Here's how the part is built. I have some questions about the finished solid (model axes, mm). A direction names the side the tool comes from. Round coordinates to 2 decimals unless told otherwise and drop trailing zeros. Write each loop counter-clockwise with the first axis right and the second up, starting at its lowest first coordinate (ties: lowest second). Pieces come first, ordered by that corner, then holes. Notation, with made-up numbers: (6.25, 51.25) -> (27.25, 51.25) arc R20 cw to (27.25, 76.25) -> close; hole circle Ø4 at (82, 75.25). An arc over 180 degrees is marked (long way). Put each result on its own line as item: value. Start each with the question number.
1. Suppose I cut it at B-B (z = 58). Please give me the cut outline in (x, y).
2. For pin 1 (0.5 mm diameter, centred on x = 0.5, z = -26, fed in from -Y), with a flat end and sliding along its axis, tell me the tip position at first contact or that it passes through.
3. Which directions (+Z, -Z, +X, -X, +Y, -Y) give clear straight access to the entire face, cutting with the end or side of a thin tool? Please do faces 1 (the face through (0.8, 126.57, 160.9)), 2 (the face through (0.78, -10.79, 128.81)).
4. I need wall thicknesses on probe 1 along Z at (x, y) = (1.25, 8.5); probe 2 along Y at (x, z) = (0.25, -10.5); probe 3 along Y at (x, z) = (0.35, -2). Which ranges of each line are inside material? Lowest first, please. Write a range as from..to.
5. We'd pull the mould along Z, two halves only. Please class faces 3 (the face through (0.8, 200.01, 137.73)), 4 (the face through (1.588, 94, 2)), 5 (the face through (0.805, 183.13, 118.068)): +Z half, -Z half, draft (parallel to the pull), parting line (faces both ways), or undercut.
6. Suppose I cut it at C-C (y = 155). Please give me the cut outline in (x, z).
7. Suppose I cut it at A-A (x = 0.7). Count the separate pieces of the cut face and the enclosed holes in it, then the cut area to 3 significant figures.
Autodesk Inventor part; units mm, degrees
ref_plane "YZ Plane" through (0, 0, 0) normal (1, 0, 0) x (0, 1, 0)
ref_plane "XZ Plane" through (0, 0, 0) normal (0, 1, 0) x (-1, 0, 0)
ref_plane "XY Plane" through (0, 0, 0) normal (0, 0, 1) x (1, 0, 0)
sketch "Sketch1" plane through (0, 0, 0) normal (1, 0, 0) x (0, 1, 0)
  line L0 (-12.7, -177.8) -> (12.7, -177.8)
  line L1 (12.7, -177.8) -> (12.7, 177.8)
  line L2 (12.7, 177.8) -> (-12.7, 177.8)
  line L3 (-12.7, 177.8) -> (-12.7, -177.8)
  line L4 (-12.7, -177.8) -> (12.7, 177.8) construction
  line L5 (12.7, -177.8) -> (-12.7, 177.8) construction
  line L6 (12.7, -101.6) -> (12.7, 177.8)
  line L7 (12.7, 177.8) -> (25.4, 177.8)
  line L8 (25.4, 177.8) -> (25.4, -177.8)
  line L9 (25.4, -177.8) -> (12.7, -177.8)
  line L10 (12.7, -177.8) -> (12.7, 177.8)
  line L11 (25.4, 177.8) -> (203.2, 177.8)
  line L12 (203.2, 177.8) -> (203.2, -177.8)
  line L13 (203.2, -177.8) -> (25.4, -177.8)
  line L14 (25.4, -177.8) -> (25.4, 177.8)
  circle A0 centre (41.275, -161.925) radius 15.875
  circle A1 centre (187.325, -59.6597) radius 15.875
  line L15 (41.275, -161.925) -> (203.2, -48.5439)
  line L16 (41.275, -161.925) -> (238.9489, -161.925) construction
  line L17 (196.4305, -72.6637) -> (50.3805, -174.929)
  circle A2 centre (187.325, -59.6597) radius 10.9537
  circle A3 centre (41.275, -161.925) radius 10.9538
  point P0 (0, 0)
  point P1 (203.2, -59.6597)
  point P2 (41.275, -177.8)
  dimension "d7" = 31.75
  dimension "d8" = 31.75
  dimension "d0" = 25.4
  dimension "d1" = 355.6
  dimension "d4" = 12.7
  dimension "d5" = 177.8
  dimension "d6" = 355.6
  dimension "d9" = 35
  dimension "d10" = 21.9075
  dimension "d11" = 21.9075
extrude "Extrusion1" add sketch "Sketch1" along normal blind 1.5875 contours L3 L2 L1 L0 | L1 L7 L8 L9 | L8 A0 L13 | L8 L11 L12 L15 A1 A0 | A0 | L15 A1 L17 A0 | L15 A2 A1 | A1 L15 A2 | A1 L15 L12
sketch "Sketch2" plane through (1.5875, 0, 0) normal (1, 0, 0) x (0, 0, -1)
  line L0 (-177.8, -12.7) -> (177.8, -12.7)
  line L1 (-127, -12.7) -> (127, -12.7)
  line L2 (127, -12.7) -> (127, 25.4)
  line L3 (127, 25.4) -> (-127, 25.4)
  line L4 (-127, 25.4) -> (-127, -12.7)
  line L5 (-177.8, 203.2) -> (-177.8, -12.7)
  line L6 (177.8, -12.7) -> (177.8, 41.275)
  point P0 (0, 0)
  point P1 (127, -12.7)
  dimension "d14" = 38.1
  dimension "d15" = 50.8
  dimension "d16" = 50.8
extrude "Extrusion2" cut sketch "Sketch2" against normal blind 1.5875
sketch "Sketch3" plane through (1.5875, 0, 0) normal (1, 0, 0) x (0, 0, -1)
  line L0 (-177.8, 203.2) -> (-177.8, -12.7)
  line L1 (-177.8, -12.7) -> (-177.8, 63.5)
  line L2 (-177.8, 63.5) -> (-140.3675, 203.2)
  line L3 (59.6597, 203.2) -> (-177.8, 203.2)
  circle A0 centre (-128.1862, 187.325) radius 15.875
  circle A1 centre (-128.1862, 187.325) radius 10.9537
  point P0 (0, 0)
  point P1 (-143.5203, 191.4338)
  point P2 (-128.1862, 203.2)
  dimension "d19" = 76.2
  dimension "d20" = 165
  dimension "d23" = 31.75
  dimension "d24" = 21.9075
extrude "Extrusion3" cut sketch "Sketch3" against normal blind 1.5875 contours L3 L2 L0 | L3 A0 L2 | A1
fillet "Fillet1" radius 6.35 6 edges at (0.7937, -12.7, 127) (0.7937, -12.7, 177.8) (0.7937, 25.4, 127) (0.7937, 25.4, -127) (0.7937, -12.7, -127) (0.7937, -12.7, -177.8)
sketch "Sketch4" plane through (1.5875, 0, 0) normal (1, 0, 0) x (0, 0, -1)
  point P0 (0, 0)
sketch "Sketch5" plane through (1.5875, 0, 0) normal (1, 0, 0) x (0, 0, -1)
  circle A0 centre (59.6597, 187.325) radius 10.9537
  circle A1 centre (59.6597, 187.325) radius 25.4
  circle A2 centre (161.925, 41.275) radius 10.9538
  circle A3 centre (161.925, 41.275) radius 25.4
  circle A4 centre (26.7321, 198.9667) radius 9.525
  circle A5 centre (26.7321, 198.9667) radius 4.2333
  line L0 (59.6597, 203.2) -> (-128.1862, 203.2)
  circle A6 centre (26.7321, 198.9667) radius 2.159
  point P0 (0, 0)
  dimension "d26" = 50.8
  dimension "d27" = 50.8
  dimension "d28" = 19.05
  dimension "d29" = 8.4667
  dimension "d30" = 4.318
extrude "Extrusion4" cut sketch "Sketch5" against normal blind 1.5875 contours A6
pattern_linear "Rectangular Pattern1" count 6 spacing 25.4 along (0, 0, 1) of "Extrusion4"
properties part number "side 1.1" material "Acetal Resin, Black"
Verdict:
1. outline: (0, 25.4) -> (1.59, 25.4) -> (1.59, 203.2) -> (0, 203.2) -> close
2. pin 1: stops at y = 25.4
3. face 1: +Z, +X, -X, +Y
3. face 2: +X, -X, -Y
4. probe 1: z = -177.8..-127, 127..177.8
4. probe 2: y = 25.4..203.2
4. probe 3: y = 25.4..196.91, 201.02..203.2
5. face 3: +Z half
5. face 4: draft
5. face 5: undercut
6. outline: (0, -101.67) -> (1.59, -101.67) -> (1.59, 153.28) -> (0, 153.28) -> close
7. separate pieces: 1
7. enclosed holes: 9
7. area: 54,600 mm^2
